The model under review builds one solid part; all positions refer to its coordinate system, in mm. Face numbers are marked on the shaded views. A direction names the side the tool comes from. Give positions to 0.01 mm unless a question says otherwise; leave off trailing zeros. Loops run counter-clockwise (first coordinate to the right, second up) from the corner with the lowest first, then second, coordinate; pieces in that order, holes last. Notation, with made-up numbers: M 20.5,17 L 35.5,17 A35 cw 35.5,49 Z; hole C 76.25,-31 d2. An arc over 180 degrees is marked long. One line per item, written item: value. Start each with the question number.
Q1. We need section A-A on y = 122. Write out the cut boundary in (x, z).
Q2. We need section D-D on y = 127. Write out the cut boundary in (x, z), plus the area to 3 significant figures.
Q3. We need section C-C on x = 82.5. Write out the cut boundary in (y, z).
Q4. For pin 1 (2 mm diameter, centred on y = 127.5, z = 212.5, fed in from +X); pin 2 (4 mm diameter, centred on x = 82, y = 127, fed in from -Z); pin 3 (5 mm diameter, centred on y = 128.5, z = 212.5, fed in from -X), all flat-tipped, find the tip position at first contact; note any pin that passes through.
Q5. We need section B-B on z = 211. Write out the cut boundary in (x, y), plus the area to 3 significant figures.
Q6. For the marked faces 1, 2 and 3, list the 3-axis set-ups (+Z, -Z, +X, -X, +Y, -Y) from which the entire face can be reached by the end or side of a thin tool; tool diameter is ignored.
Q7. Mouldability with a two-part tool opening along Z and no side actions: class the marked faces 4, 5, 6 and 7 as released by +Z, released by -Z, zero draft, split by the parting line, or undercut.
Q8. To check wall thickness, follow line 1 along X through (y, z) = (125, 212.25); line 2 along Z through (x, y) = (87, 123.75); line 3 along Z through (x, y) = (82, 121.25). State the ranges of each line that lie inside material, in increasing order. Write a range as from..to.
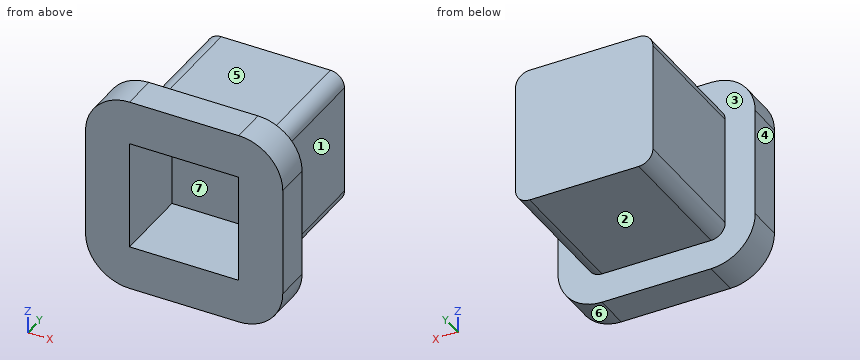
```python
from build123d import *

# Parameters (mm, degrees)
BOSS_EXTRUDE1_START = 1
BOSS_EXTRUDE1_DEPTH = 7.5
BOSS_EXTRUDE2_DEPTH = 2
SKETCH3_W           = 6.2
SKETCH3_H           = 6.2
CUT_EXTRUDE1_DEPTH  = 4.4


with BuildPart() as part:
    # Sketch1 → Boss-Extrude1 (new body)
    with BuildSketch(Plane.XZ.offset(-123.724152422).offset(BOSS_EXTRUDE1_START)):
        with BuildLine():
            Line((80.976379089, 210.746126643), (80.976379089, 216.946126643))
            ThreePointArc((80.976379089, 216.946126643), (81.210693664, 217.511812068), (81.776379089, 217.746126643))
            Line((81.776379089, 217.746126643), (87.976379089, 217.746126643))
            ThreePointArc((87.976379089, 217.746126643), (88.542064514, 217.511812068), (88.776379089, 216.946126643))
            Line((88.776379089, 216.946126643), (88.776379089, 210.746126643))
            ThreePointArc((88.776379089, 210.746126643), (88.542064514, 210.180441218), (87.976379089, 209.946126643))
            Line((87.976379089, 209.946126643), (81.776379089, 209.946126643))
            ThreePointArc((81.776379089, 209.946126643), (81.210693664, 210.180441218), (80.976379089, 210.746126643))
        make_face()
    extrude(amount=-BOSS_EXTRUDE1_DEPTH)

    # Sketch2 → Boss-Extrude2 (add)
    with BuildSketch(Plane.XZ.offset(-122.724152422)):
        with BuildLine():
            Line((81.776379089, 208.246126643), (87.976379089, 208.246126643))
            ThreePointArc((87.976379089, 208.246126643), (89.744146042, 208.97835969), (90.476379089, 210.746126643))
            Line((90.476379089, 210.746126643), (90.476379089, 216.946126643))
            ThreePointArc((90.476379089, 216.946126643), (89.744146042, 218.713893596), (87.976379089, 219.446126643))
            Line((87.976379089, 219.446126643), (81.776379089, 219.446126643))
            ThreePointArc((81.776379089, 219.446126643), (80.008612136, 218.713893596), (79.276379089, 216.946126643))
            Line((79.276379089, 216.946126643), (79.276379089, 210.746126643))
            ThreePointArc((79.276379089, 210.746126643), (80.008612136, 208.97835969), (81.776379089, 208.246126643))
        make_face()
    extrude(amount=BOSS_EXTRUDE2_DEPTH)

    # Sketch3 → Cut-Extrude1 (cut)
    with BuildSketch(Plane.XZ.offset(-120.724152422)):
        with Locations((84.876379089, 213.846126643)):
            Rectangle(SKETCH3_W, SKETCH3_H)
    extrude(amount=-CUT_EXTRUDE1_DEPTH, mode=Mode.SUBTRACT)


solid = part.part
```
Solved:
1. outline: M 79.28,210.75 A2.5 ccw 81.78,208.25 L 87.98,208.25 A2.5 ccw 90.48,210.75 L 90.48,216.95 A2.5 ccw 87.98,219.45 L 81.78,219.45 A2.5 ccw 79.28,216.95 Z; hole M 81.78,210.75 L 87.98,210.75 L 87.98,216.95 L 81.78,216.95 Z
2. outline: M 80.98,210.75 A0.8 ccw 81.78,209.95 L 87.98,209.95 A0.8 ccw 88.78,210.75 L 88.78,216.95 A0.8 ccw 87.98,217.75 L 81.78,217.75 A0.8 ccw 80.98,216.95 Z
2. area: 60.3 mm2
3. outline: M 120.72,208.25 L 122.72,208.25 L 122.72,209.95 L 130.22,209.95 L 130.22,217.75 L 122.72,217.75 L 122.72,219.45 L 120.72,219.45 L 120.72,216.95 L 125.12,216.95 L 125.12,210.75 L 120.72,210.75 Z
4. pin 1: x = 88.78
4. pin 2: z = 209.95
4. pin 3: x = 80.98
5. outline: M 79.28,120.72 L 81.78,120.72 L 81.78,125.12 L 87.98,125.12 L 87.98,120.72 L 90.48,120.72 L 90.48,122.72 L 88.78,122.72 L 88.78,130.22 L 80.98,130.22 L 80.98,122.72 L 79.28,122.72 Z
5. area: 53.6 mm2
6. face 1: +Z, -Z, +X, +Y
6. face 2: -Z, +X, -X, +Y
6. face 3: +Y
7. face 4: zero draft
7. face 5: released by +Z
7. face 6: released by -Z
7. face 7: undercut
8. line 1: 80.98..81.78, 87.98..88.78
8. line 2: 209.95..210.75, 216.95..217.75
8. line 3: 208.25..210.75, 216.95..219.45
